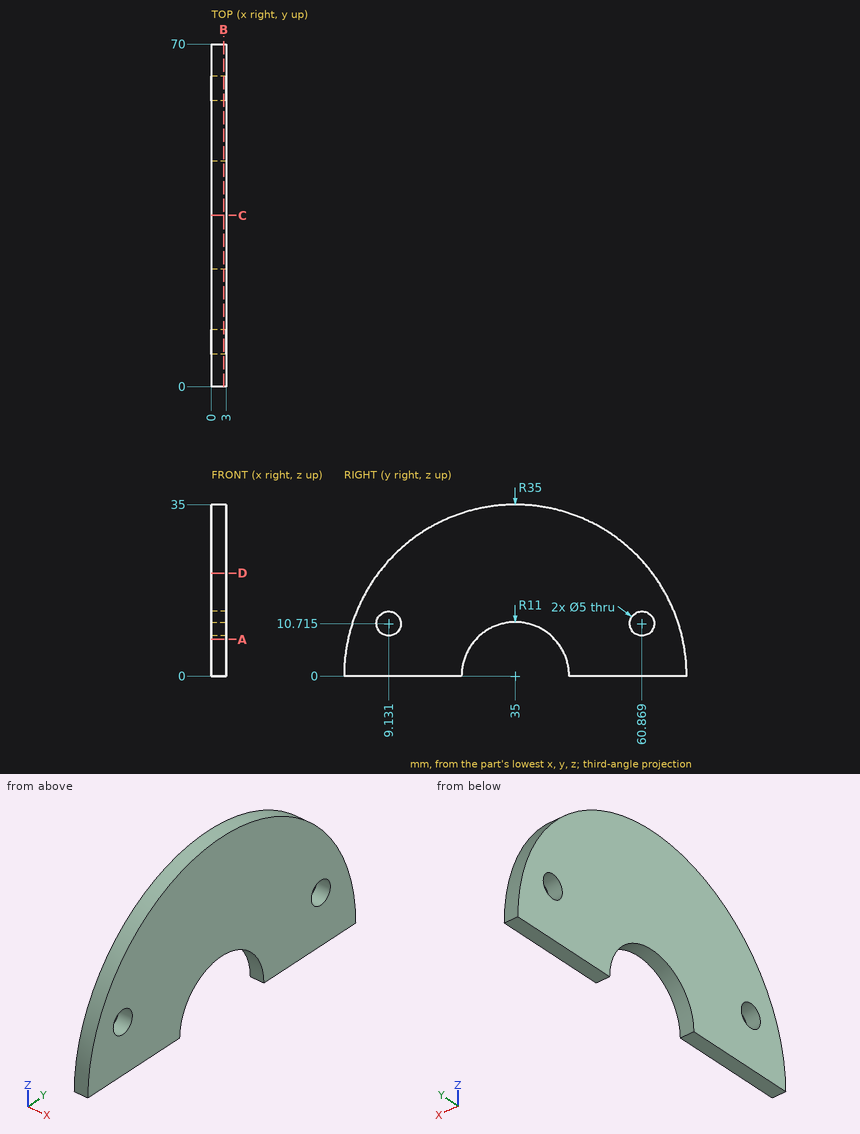
Answer from the drawing. Dimensions are ordinates in mm from the lowest x, y and z of the part. Give positions to 0.01 mm unless a question says otherwise; leave off trailing zeros. Order: outer loops, then holes, each group sorted by start corner. A loop starts at its lowest first (then second) coordinate and runs counter-clockwise, first axis right, second up. Notation, with made-up numbers: (-17.75, -17.5) -> (35.25, -17.5) arc R19 ccw to (35.25, 16.5) -> close; hole circle Ø10 at (40.25, 51). An arc over 180 degrees is marked (long way). Answer as a JSON object with one key per item and string values. Group by question number.
1. Section C-C on y = 35 is taken. Determine the outline of the cut face in (x, z), plus the area to 3 significant figures.
2. Flat-ended cylindrical pins translate along their axes: pin 1 Ø8 at (y, z) = (33, 27.5) entering from -X; pin 2 Ø1 at (x, z) = (1.5, 16) entering from -Y; pin 3 Ø4.5 at (y, z) = (9.13, 10.72) entering from -X; pin 4 Ø1.5 at (x, z) = (2.5, 31) entering from -Y (1 decimal). Find the tip coordinate at first contact, or state that the pin passes through.
3. Section D-D on z = 21 is taken. Determine the outline of the cut face in (x, y).
4. Consider line 1 along Y through (x, z) = (1, 12) (1 decimal); line 2 along Y through (x, z) = (1.1, 4); line 3 along Y through (x, z) = (2.7, 7.5) (1 decimal). Determine where each line is inside the solid, lowest interval first. Write a range as [from, to].
5. Section A-A on z = 7.5 is taken. Determine the outline of the cut face in (x, y), plus the area to 3 significant figures.
6. Section B-B on x = 2.5 is taken. Determine the outline of the cut face in (y, z) (1 decimal).
Result sheet:
{
 "1": {"outline": "(0, 11) -> (3, 11) -> (3, 35) -> (0, 35) -> close", "area": "72.0 mm^2"},
 "2": {"pin 1": "stops at x = 0", "pin 2": "stops at y = 3.62", "pin 3": "passes through", "pin 4": "stops at y = 17.4"},
 "3": {"outline": "(0, 7) -> (3, 7) -> (3, 63) -> (0, 63) -> close"},
 "4": {"line 1": "y = [2.1, 7], [11.3, 58.7], [63, 67.9]", "line 2": "y = [0.23, 24.75], [45.25, 69.77]", "line 3": "y = [0.8, 27], [43, 69.2]"},
 "5": {"outline": "(0, 0.81) -> (3, 0.81) -> (3, 26.95) -> (0, 26.95) -> close; (0, 43.05) -> (3, 43.05) -> (3, 69.19) -> (0, 69.19) -> close", "area": "157 mm^2"},
 "6": {"outline": "(0, 0) -> (24, 0) arc R11 cw to (46, 0) -> (70, 0) arc R35 ccw to start; hole circle Ø5 at (9.1, 10.7); hole circle Ø5 at (60.9, 10.7)"}
}
